Here's how the part is built. I have some questions about the finished solid (model axes, mm). Face numbers are marked on the shaded views. A direction names the side the tool comes from. Coordinates: 2 decimals unless noted, no trailing zeros. Write each loop counter-clockwise with the first axis right and the second up, starting at its lowest first coordinate (ties: lowest second). Pieces come first, ordered by that corner, then holes. Notation, with made-up numbers: M -13.75,-16 L 41.25,-16 A27 ccw 41.25,2 Z; hole C -22.75,59.5 d10. An arc over 180 degrees is marked long. Use one line per item in the form item = value. Start each with the question number.
1. Thinking about a two-plate mould opening in X: for the marked faces 3, 4 and 5, which applies, released by +X, released by -X, zero draft, split by the parting line, or undercut?
2. Please list where these lines run through material, in increasing order: line 1 along X through (y, z) = (8.25, 0); line 2 along X through (y, z) = (2, -0.5); line 3 along Z through (x, y) = (-38, 1.75). Write a range as [from, to].
3. I want a section at D-D, the plane y = 11.5. List the corners of the cut face in (x, z) for me.
4. I want a section at C-C, the plane z = -8.5. List the corners of the cut face in (x, y) for me.
5. On a 3-axis mill with a long thin cutter (end or side, diameter ignored), from which of +Z, -Z, +X, -X, +Y, -Y can I reach the whole of each face in a straight line? I mean the marked faces 1 and 2. Say none if no direction works.
6. I want a section at A-A, the plane x = -10. List the corners of the cut face in (y, z) for me.
7. I want a section at B-B, the plane y = 8. List the corners of the cut face in (x, z) for me.
8. I'm going to push flat-ended pins straight in: pin 1 Ø4 at (x, z) = (-18.5, -6) entering from +Y; pin 2 Ø0.6 at (y, z) = (0.5, 0.5) entering from -X; pin 3 Ø4 at (y, z) = (3, -5.5) entering from -X; pin 4 Ø4.5 at (x, z) = (-10, 0) entering from +Y. Where does each tip first touch, or does it pass through?
from build123d import *

# Parameters (mm, degrees)
SKETCH1_W           = 35
SKETCH1_H           = 20
SKETCH1_R           = 2.5
BOSS_EXTRUDE1_DEPTH = 10
BOSS_EXTRUDE2_DEPTH = 6.5
SKETCH3_R           = 7.5
CUT_EXTRUDE1_DEPTH  = 7
SKETCH4_R           = 2.25
CUT_EXTRUDE2_DEPTH  = 49.872282533
CHAMFER1_SIZE       = 4


with BuildPart() as part:
    # Sketch1 → Boss-Extrude1 (new body)
    with BuildSketch(Plane(origin=(0, 0, 0), x_dir=(1, 0, 0), z_dir=(0, 1, 0))):
        with Locations((-17.5, 0)):
            Rectangle(SKETCH1_W, SKETCH1_H)
        with Locations(Location((-10, 0, 0), (0, 0, 270))):
            Circle(SKETCH1_R, mode=Mode.SUBTRACT)
        with Locations(Location((-25, 0, 0), (0, 0, 270))):
            Circle(SKETCH1_R, mode=Mode.SUBTRACT)
    extrude(amount=BOSS_EXTRUDE1_DEPTH)

    # Sketch2 → Boss-Extrude2 (add)
    with BuildSketch(Plane.XY.offset(10)):
        with BuildLine():
            Line((-35, 0), (-36.778174593, 0))
            Line((-36.778174593, 0), (-40.889087297, 4.110912703))
            ThreePointArc((-40.889087297, 4.110912703), (-35.871686573, 13.383020417), (-35, 2.876524617))
            Line((-35, 2.876524617), (-35, 0))
        make_face()
    boss_extrude2 = extrude(amount=-BOSS_EXTRUDE2_DEPTH)

    # Mirror1: Boss-Extrude2 across plane
    add(boss_extrude2.mirror(Plane.XY))

    # Sketch3 → Cut-Extrude1 (cut)
    with BuildSketch(Plane.XY.offset(-3.5)):
        with Locations((-37, 8)):
            Circle(SKETCH3_R)
    extrude(amount=CUT_EXTRUDE1_DEPTH, mode=Mode.SUBTRACT)

    # Sketch4 → Cut-Extrude2 (cut, through all)
    with BuildSketch(Plane.XY.offset(10)):
        with Locations((-37, 8)):
            Circle(SKETCH4_R)
    extrude(amount=-CUT_EXTRUDE2_DEPTH, mode=Mode.SUBTRACT)

    # Chamfer1
    chamfer1_edges = [part.edges().sort_by_distance(p)[0] for p in [
        (0, 5, -10),
        (0, 5, 10),
    ]]
    chamfer(chamfer1_edges, length=CHAMFER1_SIZE)


solid = part.part
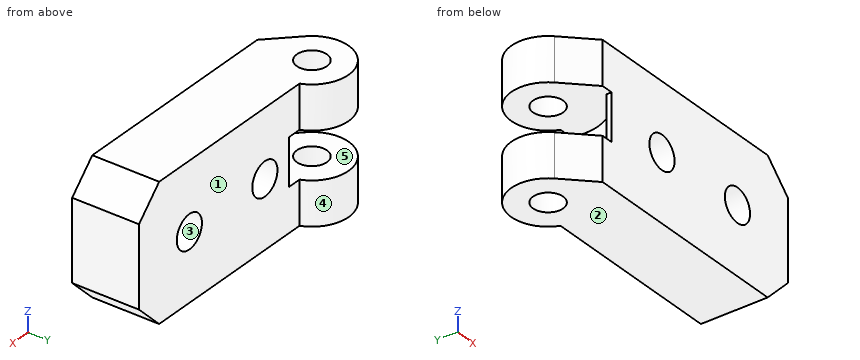
Answer list:
q1.face_3 = undercut
q1.face_4 = split by the parting line
q1.face_5 = zero draft
q2.line_1 = [-29.5, -27.5], [-22.5, -12.5], [-7.5, 0]
q2.line_2 = [-32.5, -27.45], [-22.55, -12.45], [-7.55, 0]
q2.line_3 = [-10, -3.5], [3.5, 10]
q3.outline = M -41.24,-10 L -32.76,-10 L -32.76,-3.5 L -41.24,-3.5 Z; M -41.24,3.5 L -32.76,3.5 L -32.76,10 L -41.24,10 Z
q4.outline = M -40.89,4.11 L -36.78,0 L -2.5,0 L -2.5,10 L -31.88,10 A5.5 ccw long Z; hole C -37,8 d4.5
q5.face_1 = +Z, -Z, +X, +Y
q5.face_2 = -Z, +X, -X, +Y, -Y
q6.outline = M 0,-10 L 10,-10 L 10,-2.5 L 0,-2.5 Z; M 0,2.5 L 10,2.5 L 10,10 L 0,10 Z
q7.outline = M -42.5,-10 L -39.25,-10 L -39.25,-3.5 L -42.5,-3.5 Z; M -42.5,3.5 L -39.25,3.5 L -39.25,10 L -42.5,10 Z; M -34.75,-10 L -4,-10 L 0,-6 L 0,6 L -4,10 L -34.75,10 L -34.75,3.5 L -29.5,3.5 L -29.5,-3.5 L -34.75,-3.5 Z; hole C -25,0 d5; hole C -10,0 d5
q8.pin_1 = 10
q8.pin_2 = -35
q8.pin_3 = -41.61
q8.pin_4 = through
